Here's how the part is built. I have some questions about the finished solid (model axes, mm). Face numbers are marked on the shaded views. A direction names the side the tool comes from. Coordinates: 2 decimals unless noted, no trailing zeros. Write each loop counter-clockwise with the first axis right and the second up, starting at its lowest first coordinate (ties: lowest second). Pieces come first, ordered by that corner, then holes. Notation, with made-up numbers: (78.25, 29.5) -> (107.25, 29.5) arc R21 cw to (107.25, 58.5) -> close; hole circle Ø3 at (64, 68). An arc over 180 degrees is marked (long way). Put each result on its own line as item: value. Start each with the question number.
Item 1: For pin 1 (0.8 mm diameter, centred on x = 0.5, y = 0.5, fed in from +Z); pin 2 (6.5 mm diameter, centred on x = 0.5, y = -0.5, fed in from +Z) (3 decimals); pin 3 (4 mm diameter, centred on x = -11.5, y = 1, fed in from +Z) (3 decimals); pin 4 (1 mm diameter, centred on x = 0.5, z = 16.5, fed in from -Y), each with a flat end and sliding along its axis, tell me the tip position at first contact or that it passes through.
Item 2: If we mould it in two halves opening along Y, with no side actions, what happens to the marked faces 1, 2, 3 and 4? For each: released by +Y, released by -Y, zero draft, split by the parting line, or undercut.
Item 3: I want a section at B-B, the plane z = -1. List the corners of the cut face in (x, y) for me.
Item 4: On a 3-axis mill with a long thin cutter (end or side, diameter ignored), from which of +Z, -Z, +X, -X, +Y, -Y can I reach the whole of each face in a straight line? I mean the marked faces 5, 6, 7, 8 and 9. Say none if no direction works.
Item 5: I need wall thicknesses on line 1 (X direction, y = 0, z = -1.8); line 2 (X direction, y = 3.75, z = 2.75); line 3 (Y direction, x = 0, z = 15). Which ranges of each line are inside material? Lowest first, please. Write a range as [from, to].
Item 6: I want a section at D-D, the plane y = 0. State how many separate pieces and enclosed holes the cut face has, then the cut area to 3 significant figures.
Item 7: I want a section at A-A, the plane x = -19.05. List the corners of the cut face in (y, z) for me (3 decimals).
from build123d import *

# Parameters (mm, degrees)
F1_DEPTH       = 6.35
F3_D           = 4.4958
F3_CSINK_D     = 9.1186
F3_CSINK_ANGLE = 82


with BuildPart() as f1:
    # F0 (on Front) → F1 (new body, symmetric)
    with BuildSketch(Plane.XZ):
        Polygon((25.4, -3.175), (25.4, 3.175), (12.7, 3.175), (6.35, 9.525), (-6.35, 9.525), (-12.7, 3.175), (-25.4, 3.175), (-25.4, -3.175), align=None)
    extrude(amount=F1_DEPTH, both=True)

    # F3 (through all)
    with Locations(Plane.XY.offset(3.175)):
        with Locations((-19.05, 0), (19.05, 0)):
            CounterSinkHole(F3_D / 2, F3_CSINK_D / 2, counter_sink_angle=F3_CSINK_ANGLE)

    # F4 (on Front) → F5 (revolve)
    with BuildSketch(Plane.XZ):
        Polygon((0, 12.7), (0, 9.525), (4.7625, 9.525), (4.7625, 12.7), (1.5875, 14.5330871047), (1.5875, 21.0544564477), (3.175, 21.971), (3.175, 22.225), (1.3335, 21.1618094793), (1.3335, 12.7), align=None)
    revolve(axis=Axis((0, 0, 11.1125), (0, 0, 1)))


solid = f1.part
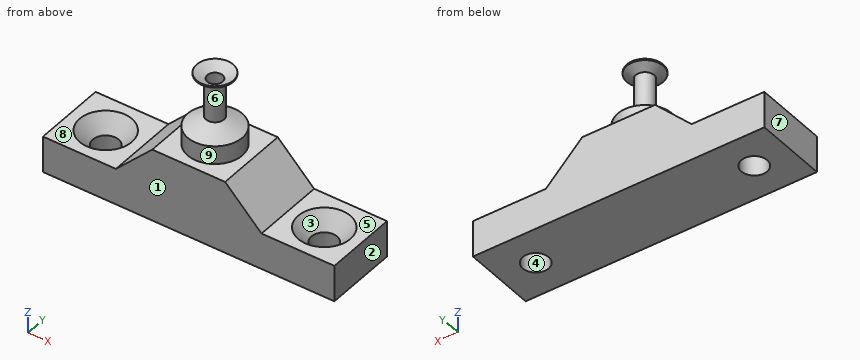
Calculated:
1. pin 1: stops at z = 12.7
1. pin 2: stops at z = 22.225
1. pin 3: stops at z = 6.375
1. pin 4: stops at y = -1.59
2. face 1: released by -Y
2. face 2: zero draft
2. face 3: undercut
2. face 4: undercut
3. outline: (-25.4, -6.35) -> (25.4, -6.35) -> (25.4, 6.35) -> (-25.4, 6.35) -> close; hole circle Ø4.5 at (-19.05, 0); hole circle Ø4.5 at (19.05, 0)
4. face 5: +Z, +X, +Y, -Y
4. face 6: none
4. face 7: +Z, -Z, -X, +Y, -Y
4. face 8: +Z, -X, +Y, -Y
4. face 9: +Z
5. line 1: x = [-25.4, -21.3], [-16.8, 16.8], [21.3, 25.4]
5. line 2: x = [-25.4, -20.92], [-17.18, 17.18], [20.92, 25.4]
5. line 3: y = [-1.59, -1.33], [1.33, 1.59]
6. separate pieces: 3
6. enclosed holes: 0
6. area: 415 mm2
7. outline: (-6.35, -3.175) -> (-2.248, -3.175) -> (-2.248, 0.516) -> (-4.559, 3.175) -> (-6.35, 3.175) -> close; (2.248, -3.175) -> (6.35, -3.175) -> (6.35, 3.175) -> (4.559, 3.175) -> (2.248, 0.516) -> close
